Work out the finished part from the listing and answer in its coordinate system (mm). Round coordinates to 2 decimals unless told otherwise and drop trailing zeros. Loops run counter-clockwise (first coordinate to the right, second up) from the corner with the lowest first, then second, coordinate; pieces in that order, holes last. Notation, with made-up numbers: (61.25, 36) -> (116.25, 36) arc R15 ccw to (116.25, 52) -> close; hole circle Ø6 at (-30, 75.25). An arc over 180 degrees is marked (long way). Use CSV: the item, a comma, the result in double quotes. Start each with the question number.
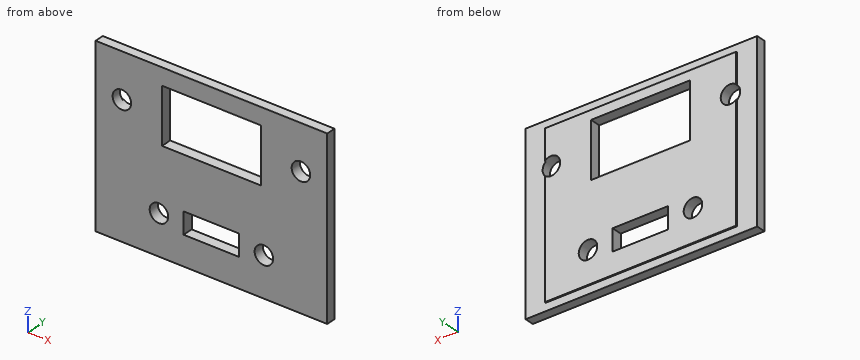
Autodesk Inventor part; units mm, degrees
ref_plane "YZ Plane" through (0, 0, 0) normal (1, 0, 0) x (0, 1, 0)
ref_plane "XZ Plane" through (0, 0, 0) normal (0, 1, 0) x (-1, 0, 0)
ref_plane "XY Plane" through (0, 0, 0) normal (0, 0, 1) x (1, 0, 0)
sketch "Sketch1" plane through (0, 0, 0) normal (0, 1, 0) x (-1, 0, 0)
  line L0 (15.5, 13) -> (-15.5, 13)
  line L1 (-15.5, 13) -> (-15.5, -13)
  line L2 (-15.5, -13) -> (15.5, -13)
  line L3 (15.5, -13) -> (15.5, 13)
  line L4 (15.5, 13) -> (-15.5, -13) construction
  line L5 (-15.5, 13) -> (15.5, -13) construction
  line L6 (18.75, -14.25) -> (-18.75, -14.25)
  line L7 (-18.75, -14.25) -> (-18.75, 14.25)
  line L8 (-18.75, 14.25) -> (18.75, 14.25)
  line L9 (18.75, 14.25) -> (18.75, -14.25)
  line L10 (18.75, -14.25) -> (-18.75, 14.25) construction
  line L11 (-18.75, -14.25) -> (18.75, 14.25) construction
  point P0 (0, 0)
  dimension "d0" = 31
  dimension "d1" = 26
  dimension "d16" = 37.5
  dimension "d17" = 28.5
extrude "Extrusion2" add sketch "Sketch1" along normal blind 1.5 contours L3 L2 L1 L0 | L6 L7 L8 L9
sketch "Sketch2" plane through (0, 1.5, 0) normal (0, 1, 0) x (1, 0, 0)
  line L0 (15.5, 13) -> (-15.5, 13)
  line L1 (-15.5, -13) -> (15.5, -13)
  line L2 (-18.75, -14.25) -> (18.75, -14.25)
  line L3 (18.75, -14.25) -> (18.75, 14.25)
  line L4 (18.75, 14.25) -> (-18.75, 14.25)
  line L5 (-18.75, 14.25) -> (-18.75, -14.25)
  line L6 (15.5, -13) -> (15.5, 13)
  line L7 (-15.5, 13) -> (-15.5, -13)
  point P0 (0, 0)
extrude "Extrusion4" add sketch "Sketch2" along normal blind 0.2 contours L6 L1 L7 L0
sketch "Sketch3" plane through (0, 1.7, 0) normal (0, 1, 0) x (1, 0, 0)
  circle A0 centre (-14.5, -7) radius 1.5
  circle A1 centre (14.5, -7) radius 1.5
  circle A2 centre (-8.5, 7.75) radius 1.5
  circle A3 centre (8.5, 7.75) radius 1.5
  line L0 (0, -13.0822) -> (0, 13.0822)
  line L1 (-15.5, -13) -> (15.5, -13)
  line L2 (15.5, 13) -> (-15.5, 13)
  line L3 (8, -11.5) -> (-8, -11.5)
  line L4 (-8, -11.5) -> (-8, -2.5)
  line L5 (-8, -2.5) -> (8, -2.5)
  line L6 (8, -2.5) -> (8, -11.5)
  line L7 (8, -11.5) -> (-8, -2.5) construction
  line L8 (-8, -11.5) -> (8, -2.5) construction
  line L9 (4.5, 6) -> (-4.5, 6)
  line L10 (-4.5, 6) -> (-4.5, 9.5)
  line L11 (-4.5, 9.5) -> (4.5, 9.5)
  line L12 (4.5, 9.5) -> (4.5, 6)
  line L13 (4.5, 6) -> (-4.5, 9.5) construction
  line L14 (-4.5, 6) -> (4.5, 9.5) construction
  point P0 (0, 0)
  point P1 (0, -7)
  point P2 (0, 7.75)
  dimension "d25" = 3
  dimension "d26" = 3
  dimension "d27" = 3
  dimension "d28" = 3
  dimension "d29" = 8.5
  dimension "d30" = 8.5
  dimension "d31" = 14.5
  dimension "d32" = 14.5
  dimension "d33" = 6
  dimension "d34" = 6
  dimension "d35" = 5.25
  dimension "d36" = 5.25
  dimension "d37" = 16
  dimension "d38" = 9
  dimension "d39" = 9
  dimension "d40" = 3.5
extrude "Extrusion5" cut sketch "Sketch3" against normal up to surface (1.7 mm away)
sketch "Sketch4" plane through (0, 0, 0) normal (0, -1, 0) x (1, 0, 0)
  line L0 (-15.5, 13) -> (15.5, 13)
  line L1 (15.5, 13) -> (15.5, -13)
  line L2 (-15.5, -13) -> (-15.5, 13)
  line L3 (15.5, -13) -> (-15.5, -13)
  point P0 (0, 0)
equation "\"d30\" = d29"
equation "\"d32\" = d31"
equation "\"d34\" = d33"
equation "\"d36\" = d35"
properties part number "USB inner clamp plate_3DPrint"
Q1. Straight lines are drawn through the part: line 1 (X direction, y = 0.5, z = 7); line 2 (X direction, y = 0.75, z = -7.75); line 3 (X direction, y = 0.4, z = 9.25). For each, find the intervals that lie inside material, in ascending order. Write a range as from..to.
Q2. Section D-D, the plane x = -8.5 is taken. Write down the section's boundary in (y, z).
Q3. Section C-C, the plane z = 4 is taken. Write down the section's boundary in (x, y), and give its area (4 significant figures).
Q4. Section B-B, the plane z = 7 is taken. Write down the section's boundary in (x, y).
Q5. Section A-A, the plane x = -2 is taken. Write down the section's boundary in (y, z), and give its area (3 significant figures).
Q6. This flat-tipped pin is pushed along its axis until it touches: pin 1 (4 mm diameter, centred on x = -14.5, z = 7, fed in from -Y). Where does it stop, or does it pass through?
Report:
1,line 1,"x = -18.75..-16, -13..-8, 8..13, 16..18.75"
1,line 2,"x = -18.75..-10, -7..-4.5, 4.5..7, 10..18.75"
1,line 3,"x = -18.75..-8, 8..18.75"
2,outline,"(0, -14.25) -> (1.5, -14.25) -> (1.5, -13) -> (1.7, -13) -> (1.7, -9.25) -> (0, -9.25) -> close; (0, -6.25) -> (1.7, -6.25) -> (1.7, 13) -> (1.5, 13) -> (1.5, 14.25) -> (0, 14.25) -> close"
3,outline,"(-18.75, 0) -> (-8, 0) -> (-8, 1.7) -> (-15.5, 1.7) -> (-15.5, 1.5) -> (-18.75, 1.5) -> close; (8, 0) -> (18.75, 0) -> (18.75, 1.5) -> (15.5, 1.5) -> (15.5, 1.7) -> (8, 1.7) -> close"
3,area,"35.25 mm²"
4,outline,"(-18.75, 0) -> (-16, 0) -> (-16, 1.5) -> (-18.75, 1.5) -> close; (-13, 0) -> (-8, 0) -> (-8, 1.7) -> (-13, 1.7) -> close; (8, 0) -> (13, 0) -> (13, 1.7) -> (8, 1.7) -> close; (16, 0) -> (18.75, 0) -> (18.75, 1.5) -> (16, 1.5) -> close"
5,outline,"(0, -14.25) -> (1.5, -14.25) -> (1.5, -13) -> (1.7, -13) -> (1.7, -9.5) -> (0, -9.5) -> close; (0, -6) -> (1.7, -6) -> (1.7, 2.5) -> (0, 2.5) -> close; (0, 11.5) -> (1.7, 11.5) -> (1.7, 13) -> (1.5, 13) -> (1.5, 14.25) -> (0, 14.25) -> close"
5,area,"26.7 mm²"
6,pin 1,"stops at y = 0"
